Geometry check sheet. Reference: the model listing, model coordinates, mm. A direction names the side the tool comes from. Give positions to 0.01 mm unless a question says otherwise; leave off trailing zeros. Write each loop counter-clockwise with the first axis right and the second up, starting at its lowest first coordinate (ties: lowest second). Pieces come first, ordered by that corner, then holes. Notation, with made-up numbers: (18.5, 12.25) - (35.5, 12.25) arc R27 ccw to (35.5, 51.25) - close; hole circle Ø1 at (-30.5, -1.5). An arc over 180 degrees is marked (long way). Write item = value, one per line. Start each with the question number.
(1) Access from +Z, -Z, +X, -X, +Y, -Y to the whole of each face (thin tool, end or side, straight path). Record for faces 3 (the cylindrical face through (-5.621, 37.444, 2.958)), 4 (the flat face through (-21.299, 48, 3)).
(2) Thickness scan on L1, parallel to X at y = 27.5, z = 4.95; L2, parallel to Y at x = -24.5, z = 1.4; L3, parallel to X at y = 4, z = 4. Record the ranges inside material, lowest first.
(3) Draft check along X on faces 1 (the cylindrical face through (-33.59, 4.32, 2.96)), 2 (the flat face through (-13, 19, 0)). Enter one of: pulls with the +X half, pulls with the -X half, needs draft (parallel to the pull), parting line crosses it, or undercut.
(4) Section check A-A, the plane y = 32. Enter the section's corners in (x, z).
(5) Section check B-B, the plane x = -27.5. Enter the section's corners in (y, z), plus the area to 3 significant figures.
(6) Section check C-C, the plane x = -39.5. Enter the section's corners in (y, z).
(7) Depth check by flat-ended pin: pin 1 Ø12 at (x, y) = (-4.74, 30.7) entering from +Z; pin 2 Ø1.5 at (y, z) = (38, 5) entering from -X. Enter the tip coordinate at first touch or a pass-through.
(8) Section check D-D, the plane z = 4.5. Give the number of separate pieces and of enclosed holes in the cut face, plus the area to 3 significant figures.
```python
from build123d import *

# Parameters (mm, degrees)
SZKIC1_R                    = 6.5
SZKIC1_R_2                  = 4.5
SZKIC1_R_3                  = 6.800419073
DODANIE_WYCI_GNI_CIE1_DEPTH = 6


with BuildPart() as part:
    # Szkic1 → Dodanie-wyciągnięcie1 (new body)
    with BuildSketch(Plane.XY):
        with BuildLine():
            ThreePointArc((10.70117022, 18.531289035), (2.291892255, 39.56102988), (-18.29882978, 48.994381459))
            Line((-18.29882978, 48.994381459), (-18.29882978, 47.631289035))
            ThreePointArc((-18.29882978, 47.631289035), (-19.79882978, 46.131289035), (-21.29882978, 47.631289035))
            Line((-21.29882978, 47.631289035), (-21.29882978, 48.994381459))
            ThreePointArc((-21.29882978, 48.994381459), (-40.828570624, -3.559432999), (10.70117022, 18.531289035))
        make_face()
        with Locations((-37.156723858, 16.008369355)):
            Circle(SZKIC1_R, mode=Mode.SUBTRACT)
        with Locations((-27.094885778, 4.029990689)):
            Circle(SZKIC1_R, mode=Mode.SUBTRACT)
        with Locations((-10.964002507, 4.029990689)):
            Circle(SZKIC1_R, mode=Mode.SUBTRACT)
        with Locations((-19.79882978, 18.531289035)):
            Circle(SZKIC1_R_2, mode=Mode.SUBTRACT)
        with Locations((-2.020146436, 16.008369355)):
            Circle(SZKIC1_R, mode=Mode.SUBTRACT)
        with Locations((-35.240183271, 30.701847186)):
            Circle(SZKIC1_R, mode=Mode.SUBTRACT)
        with Locations((-4.7352456, 30.701847186)):
            Circle(SZKIC1_R_3, mode=Mode.SUBTRACT)
        with Locations((-19.797413553, 36.031288978)):
            Circle(SZKIC1_R, mode=Mode.SUBTRACT)
    extrude(amount=DODANIE_WYCI_GNI_CIE1_DEPTH)


solid = part.part
```
Model answer:
q1.face_3 = +Z, -Z
q1.face_4 = +Z, -Z, +Y
q2.L1 = -48.95 to -40.9, -29.58 to -10.73, 1.26 to 9.35
q2.L2 = -11.6 to -1.93, 9.99 to 31.54, 40.52 to 48.67
q2.L3 = -46.61 to -33.59, -20.59 to -17.46, -4.46 to 7.02
q3.face_1 = undercut
q3.face_2 = needs draft
q4.outline = (-47.16, 0) - (-41.61, 0) - (-41.61, 6) - (-47.16, 6) - close; (-28.87, 0) - (-24.9, 0) - (-24.9, 6) - (-28.87, 6) - close; (-14.7, 0) - (-11.41, 0) - (-11.41, 6) - (-14.7, 6) - close; (1.94, 0) - (7.57, 0) - (7.57, 6) - (1.94, 6) - close
q5.outline = (-10.98, 0) - (-2.46, 0) - (-2.46, 6) - (-10.98, 6) - close; (10.52, 0) - (48.04, 0) - (48.04, 6) - (10.52, 6) - close
q5.area = 276 mm²
q6.outline = (-4.75, 0) - (9.95, 0) - (9.95, 6) - (-4.75, 6) - close; (22.07, 0) - (25.79, 0) - (25.79, 6) - (22.07, 6) - close; (35.61, 0) - (41.81, 0) - (41.81, 6) - (35.61, 6) - close
q7.pin_1 = through
q7.pin_2 = -43.88
q8.separate_pieces = 1
q8.enclosed_holes = 8
q8.area = 1,910 mm²
